Can you work these out from the model? Positions are in its coordinate system, mm. A direction names the side the tool comes from. Round coordinates to 2 decimals unless told otherwise and drop trailing zeros. Write each loop counter-clockwise with the first axis right and the second up, starting at its lowest first coordinate (ties: lowest second). Pieces come first, ordered by that corner, then holes. Notation, with made-up numbers: M 74,28.5 L 80,28.5 A18 cw 80,41.5 Z; hole C 49,-21.5 d6. An arc over 180 degrees is marked long. Answer in a Markdown table with one row per item. Add a question column.
(1) If we mould it in two halves opening along X, with no side actions, what happens to faces 1 (the face through (-117.457, 0.654, 7.243)), 2 (the face through (-2, 46.736, 14)), 3 (the face through (115.04, -56.22, 93.64)), 4 (the face through (125.095, -1, 61))? For each: released by +X, released by -X, zero draft, split by the parting line, or undercut.
(2) I'm going to push flat-ended pins straight in: pin 1 (1 mm diameter, centred on x = -2.5, y = 34.5, fed in from +Z) (3 decimals); pin 2 (12.5 mm diameter, centred on x = 117.16, y = -59.54, fed in from -Z) (3 decimals); pin 3 (4.5 mm diameter, centred on x = -117.16, y = 59.54, fed in from -Z); pin 4 (17.5 mm diameter, centred on x = 116.5, y = -58, fed in from -Z). Where does each tip first touch, or does it pass through?
(3) Suppose I cut it at C-C, the plane x = 61. Write out the boundary of the cut face in (y, z) (3 decimals), then the cut area to 3 significant figures.
(4) Suppose I cut it at B-B, the plane y = 10.5. Write out the boundary of the cut face in (x, z) (3 decimals), then the cut area to 3 significant figures.
(5) Suppose I cut it at A-A, the plane z = 35.5. Write out the boundary of the cut face in (x, y) (3 decimals).
(6) If I drill on probe 1 along X at (y, z) = (-14, 76) (3 decimals); probe 2 along Z at (x, y) = (1.5, 26) (3 decimals); probe 3 along X at (y, z) = (38, 18), over which ranges is the centre line in solid material (lowest first)?
(7) For faces 5 (the face through (106.16, 0.65, 18.77)), 6 (the face through (-117, -64, 92.075)), 7 (the face through (117, 1, 95.25)), which set-ups out of +Z, -Z, +X, -X, +Y, -Y let a thin tool reach every point of the face, with its end or its side?
(8) Suppose I cut it at D-D, the plane z = 6. Write out the boundary of the cut face in (x, y).
from build123d import *

# Parameters (mm, degrees)
SKETCH1_W           = 250.19
SKETCH1_H           = 93.472
BOSS_EXTRUDE1_DEPTH = 95.25
SKETCH5_W           = 218.44
SKETCH5_H           = 93.472
CUT_EXTRUDE1_DEPTH  = 79.375
SKETCH6_W           = 15.875
SKETCH6_H           = 25.4
BOSS_EXTRUDE2_DEPTH = 3.175
SKETCH7_R           = 3.937
CUT_EXTRUDE2_DEPTH  = 172.26052419
FILLET1_R           = 25.4
FILLET2_R           = 25.4
FILLET3_R           = 5.08
FILLET4_R           = 5.08
FILLET5_R           = 5.08
FILLET6_R           = 5.08
FILLET7_R           = 10.16
FILLET8_R           = 10.16


with BuildPart() as part:
    # Sketch1 → Boss-Extrude1 (new body)
    with BuildSketch(Plane.XY):
        Rectangle(SKETCH1_W, SKETCH1_H)
    extrude(amount=BOSS_EXTRUDE1_DEPTH)

    # Sketch5 → Cut-Extrude1 (cut)
    with BuildSketch(Plane.XY.offset(95.25)):
        Rectangle(SKETCH5_W, SKETCH5_H)
    extrude(amount=-CUT_EXTRUDE1_DEPTH, mode=Mode.SUBTRACT)

    # Sketch6 → Boss-Extrude2 (add)
    with BuildSketch(Plane.XY.offset(95.25)):
        with Locations((117.1575, 59.436)):
            Rectangle(SKETCH6_W, SKETCH6_H)
        with Locations((-117.1575, 59.436)):
            Rectangle(SKETCH6_W, SKETCH6_H)
        with Locations((117.1575, -59.436)):
            Rectangle(SKETCH6_W, SKETCH6_H)
        with Locations((-117.1575, -59.436)):
            Rectangle(SKETCH6_W, SKETCH6_H)
    extrude(amount=-BOSS_EXTRUDE2_DEPTH)

    # Sketch7 → Cut-Extrude2 (cut, through all)
    with BuildSketch(Plane(origin=(0, 0, 92.075), x_dir=(-1, 0, 0), z_dir=(0, 0, -1))):
        with Locations((117.1575, 59.5376)):
            Circle(SKETCH7_R)
        with Locations(Location((-117.1575, 59.5376, 0), (0, 0, 180))):
            Circle(SKETCH7_R)
        with Locations(Location((117.1575, -59.5376, 0), (0, 0, 180))):
            Circle(SKETCH7_R)
        with Locations((-117.1575, -59.5376)):
            Circle(SKETCH7_R)
    extrude(amount=-CUT_EXTRUDE2_DEPTH, mode=Mode.SUBTRACT)

    # Fillet1
    fillet1_edges = [part.edges().sort_by_distance(p)[0] for p in [
        (125.095, 0, 0),
    ]]
    fillet(fillet1_edges, radius=FILLET1_R)

    # Fillet2
    fillet2_edges = [part.edges().sort_by_distance(p)[0] for p in [
        (-125.095, 0, 0),
    ]]
    fillet(fillet2_edges, radius=FILLET2_R)

    # Fillet3
    fillet3_edges = [part.edges().sort_by_distance(p)[0] for p in [
        (117.1575, 46.736, 92.075),
    ]]
    fillet(fillet3_edges, radius=FILLET3_R)

    # Fillet4
    fillet4_edges = [part.edges().sort_by_distance(p)[0] for p in [
        (-117.1575, 46.736, 92.075),
    ]]
    fillet(fillet4_edges, radius=FILLET4_R)

    # Fillet5
    fillet5_edges = [part.edges().sort_by_distance(p)[0] for p in [
        (-117.1575, -46.736, 92.075),
    ]]
    fillet(fillet5_edges, radius=FILLET5_R)

    # Fillet6
    fillet6_edges = [part.edges().sort_by_distance(p)[0] for p in [
        (117.1575, -46.736, 92.075),
    ]]
    fillet(fillet6_edges, radius=FILLET6_R)

    # Fillet7
    fillet7_edges = [part.edges().sort_by_distance(p)[0] for p in [
        (-109.22, 0, 15.875),
    ]]
    fillet(fillet7_edges, radius=FILLET7_R)

    # Fillet8
    fillet8_edges = [part.edges().sort_by_distance(p)[0] for p in [
        (109.22, 0, 15.875),
    ]]
    fillet(fillet8_edges, radius=FILLET8_R)


solid = part.part
Calculated:
| question | item | result |
|---|---|---|
| 1 | face 1 | released by -X |
| 1 | face 2 | zero draft |
| 1 | face 3 | undercut |
| 1 | face 4 | released by +X |
| 2 | pin 1 | z = 15.875 |
| 2 | pin 2 | z = 92.075 |
| 2 | pin 3 | through |
| 2 | pin 4 | z = 91.38 |
| 3 | outline | M -46.736,0 L 46.736,0 L 46.736,15.875 L -46.736,15.875 Z |
| 3 | area | 1,480 mm² |
| 4 | outline | M -125.095,25.4 A25.4 ccw -99.695,0 L 99.695,0 A25.4 ccw 125.095,25.4 L 125.095,95.25 L 109.22,95.25 L 109.22,26.035 A10.16 cw 99.06,15.875 L -99.06,15.875 A10.16 cw -109.22,26.035 L -109.22,95.25 L -125.095,95.25 Z |
| 4 | area | 6,260 mm² |
| 5 | outline | M -125.095,-46.736 L -109.22,-46.736 L -109.22,46.736 L -125.095,46.736 Z; M 109.22,-46.736 L 125.095,-46.736 L 125.095,46.736 L 109.22,46.736 Z |
| 6 | probe 1 | -125.095 to -109.22, 109.22 to 125.095 |
| 6 | probe 2 | 0 to 15.875 |
| 6 | probe 3 | -123.99 to -105.28, 105.28 to 123.99 |
| 7 | face 5 | +Z, +Y, -Y |
| 7 | face 6 | -Z, +X, -X, -Y |
| 7 | face 7 | +Z, +X, -X, +Y, -Y |
| 8 | outline | M -116.09,-46.74 L 116.09,-46.74 L 116.09,46.74 L -116.09,46.74 Z |
